Design review of the part built by this model. Coordinates are the model's own, in mm. A direction names the side the tool comes from. Round coordinates to 2 decimals unless told otherwise and drop trailing zeros. Write each loop counter-clockwise with the first axis right and the second up, starting at its lowest first coordinate (ties: lowest second). Pieces come first, ordered by that corner, then holes. Notation, with made-up numbers: (7.5, 44.25) -> (39.5, 44.25) arc R24 ccw to (39.5, 83.25) -> close; hole circle Ø6 at (11.25, -8). An arc over 180 degrees is marked (long way). One line per question, with ' | ' between items. Start each with the question number.
1) Consider section B-B (y = 3.5). Give the boundary of the cut face in (x, z), then the cut area to 3 significant figures.
2) Consider section C-C (x = 4.9). Give the boundary of the cut face in (y, z).
3) Mouldability with a two-part tool opening along Y and no side actions: class faces 4 (the flat face through (5, 25, 2)), 5 (the flat face through (5, 13, 0)), 6 (the flat face through (5, 13, 4.5)), 7 (the flat face through (5, 7, 7)) as +Y half, -Y half, draft (parallel to the pull), parting line (faces both ways), or undercut.
4) Consider section A-A (z = 5.25). Give the boundary of the cut face in (x, y), then the cut area to 3 significant figures.
5) Consider section D-D (y = 9.75). Give the boundary of the cut face in (x, z).
6) Insertion check: pin 1 Ø4 at (x, z) = (5.5, 7) entering from -Y; pin 2 Ø3 at (x, y) = (5.5, 4) entering from +Z; pin 3 Ø1.5 at (x, z) = (6, 3.5) entering from -Y. Each pin has a flat end and moves straight along its axis. Give the tip position at first contact, or say it passes through.
7) For probe 1 along Y at (x, z) = (4.9, 2.2); probe 2 along Y at (x, z) = (3.5, 7.5); probe 3 along Z at (x, y) = (2.5, 2), list the stretches that pass through material, from the lowest coordinate up.
8) For faces 1 (the flat face through (5, 18.7, 7)), 2 (the flat face through (1.9, 13, 4)), 3 (the flat face through (5, 11.5, 7)), list the 3-axis set-ups (+Z, -Z, +X, -X, +Y, -Y) from which the entire face can be reached by the end or side of a thin tool; tool diameter is ignored.
Autodesk Inventor part; units mm, degrees
ref_plane "YZ Plane" through (0, 0, 0) normal (1, 0, 0) x (0, 1, 0)
ref_plane "XZ Plane" through (0, 0, 0) normal (0, 1, 0) x (-1, 0, 0)
ref_plane "XY Plane" through (0, 0, 0) normal (0, 0, 1) x (1, 0, 0)
sketch "Sketch1" plane through (0, 0, 0) normal (0, 0, 1) x (1, 0, 0)
  line L0 (0, 0) -> (10.2, 0)
  line L1 (10.2, 0) -> (10.2, 25)
  line L2 (10.2, 25) -> (0, 25)
  line L3 (0, 25) -> (0, 0)
  dimension "d0" = 10.2
  dimension "d1" = 25
extrude "Extrusion1" add sketch "Sketch1" along normal blind 1.5
sketch "Sketch2" plane through (0, 0, 1.5) normal (0, 0, 1) x (1, 0, 0)
  line L0 (10.2, 0) -> (10.2, 25)
  line L1 (10.2, 25) -> (0, 25)
  line L2 (1.9, 25) -> (7.9, 25)
  line L3 (7.9, 25) -> (7.9, 0.8)
  line L4 (7.9, 0.8) -> (1.9, 0.8)
  line L5 (1.9, 0.8) -> (1.9, 25)
  dimension "d4" = 6
  dimension "d5" = 24.2
  dimension "d6" = 2.3
  dimension "d7" = 0
extrude "Extrusion2" add sketch "Sketch2" along normal blind 3
sketch "Sketch3" plane through (0, 0, 4.5) normal (0, 0, 1) x (1, 0, 0)
  line L0 (1.9, 25) -> (1.9, 0.8)
  line L1 (7.9, 0.8) -> (7.9, 25)
  line L2 (1.9, 7) -> (7.9, 7)
  line L3 (7.9, 7) -> (7.9, 11.5)
  line L4 (7.9, 11.5) -> (1.9, 11.5)
  line L5 (1.9, 11.5) -> (1.9, 7)
  line L6 (1.9, 14.4) -> (7.9, 14.4)
  line L7 (7.9, 14.4) -> (7.9, 18.7)
  line L8 (7.9, 18.7) -> (1.9, 18.7)
  line L9 (1.9, 18.7) -> (1.9, 14.4)
  line L10 (1.9, 0.8) -> (7.9, 0.8)
  point P0 (0, 0)
  dimension "d10" = 4.5
  dimension "d11" = 4.3
  dimension "d12" = 2.9
  dimension "d15" = 6.2
extrude "Extrusion3" add sketch "Sketch3" along normal blind 5.6 contours L8 L1 L6 L0 | L4 L1 L2 L0
sketch "Sketch4" plane through (0, 0, 4.5) normal (0, 0, 1) x (1, 0, 0)
  line L0 (1.9, 7) -> (1.9, 0.8)
  line L1 (1.9, 0.8) -> (7.9, 0.8)
  circle A0 centre (4.9, 3.5) radius 1.6
  line L2 (0, 25) -> (0, 0)
  dimension "d16" = 3.2
  dimension "d18" = 3
  dimension "d19" = 2.7
sketch "Sketch5" plane through (0, 0, 4.5) normal (0, 0, 1) x (1, 0, 0)
  circle A0 centre (4.9, 22.5779) radius 1.6
  circle A1 centre (4.9, 3.4779) radius 1.6
  point P0 (0, 0)
  dimension "d20" = 3.2
  dimension "d21" = 3.2
  dimension "d22" = 19.1
extrude "Extrusion4" cut sketch "Sketch5" against normal blind 5.6 contours A0
extrude "Extrusion5" cut sketch "Sketch4" against normal blind 5.6
properties part number "OptoEndStop"
From the geometry:
1) outline: (0, 0) -> (3.3, 0) -> (3.3, 4.5) -> (1.9, 4.5) -> (1.9, 1.5) -> (0, 1.5) -> close; (6.5, 0) -> (10.2, 0) -> (10.2, 1.5) -> (7.9, 1.5) -> (7.9, 4.5) -> (6.5, 4.5) -> close | area: 18.9 mm2
2) outline: (0, 0) -> (1.9, 0) -> (1.9, 4.5) -> (0.8, 4.5) -> (0.8, 1.5) -> (0, 1.5) -> close; (5.1, 0) -> (20.98, 0) -> (20.98, 4.5) -> (18.7, 4.5) -> (18.7, 10.1) -> (14.4, 10.1) -> (14.4, 4.5) -> (11.5, 4.5) -> (11.5, 10.1) -> (7, 10.1) -> (7, 4.5) -> (5.1, 4.5) -> close; (24.18, 0) -> (25, 0) -> (25, 4.5) -> (24.18, 4.5) -> close
3) face 4: +Y half | face 5: draft | face 6: undercut | face 7: -Y half
4) outline: (1.9, 7) -> (7.9, 7) -> (7.9, 11.5) -> (1.9, 11.5) -> close; (1.9, 14.4) -> (7.9, 14.4) -> (7.9, 18.7) -> (1.9, 18.7) -> close | area: 52.8 mm2
5) outline: (0, 0) -> (10.2, 0) -> (10.2, 1.5) -> (7.9, 1.5) -> (7.9, 10.1) -> (1.9, 10.1) -> (1.9, 1.5) -> (0, 1.5) -> close
6) pin 1: stops at y = 7 | pin 2: stops at z = 4.5 | pin 3: stops at y = 0.8
7) probe 1: y = 0.8 to 1.9, 5.1 to 20.98, 24.18 to 25 | probe 2: y = 7 to 11.5, 14.4 to 18.7 | probe 3: z = 0 to 4.5
8) face 1: +Z, +X, -X, +Y | face 2: +Z, -X, +Y, -Y | face 3: +Z, +X, -X
